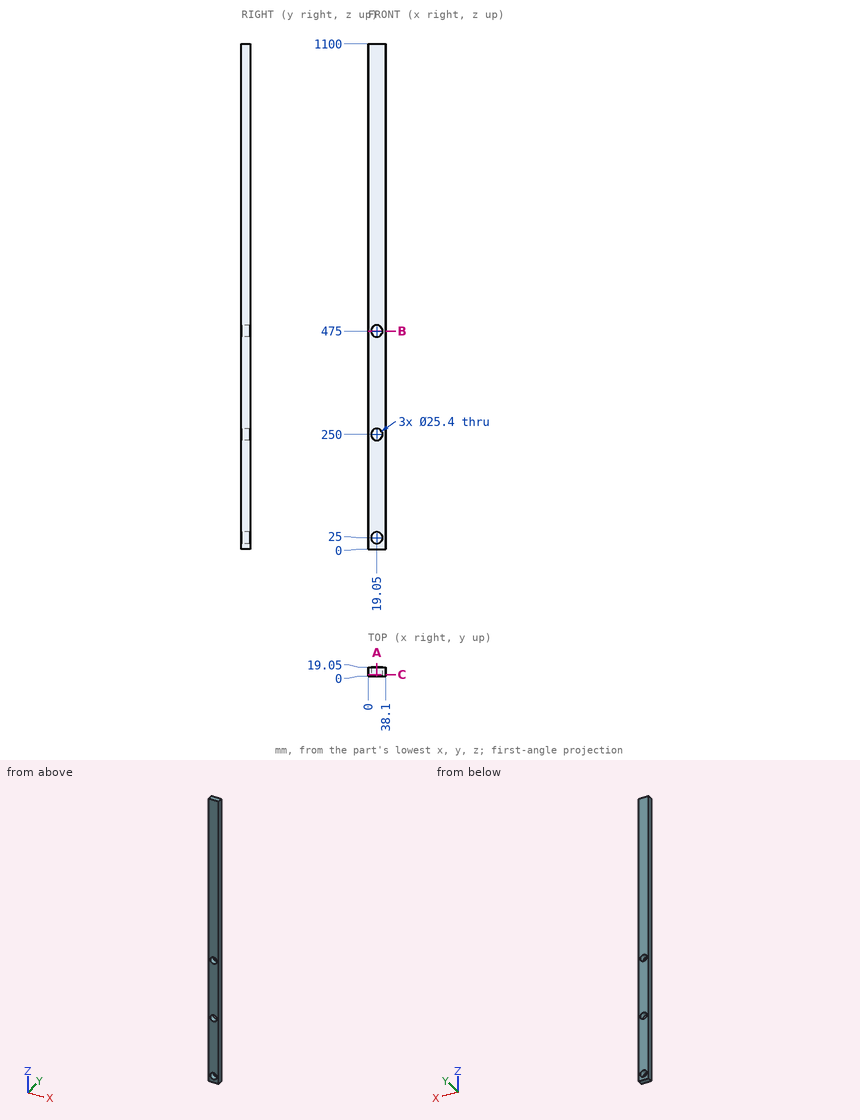
Could you check a few things on this drawing? It's one solid part, dimensions in mm from its lowest x, y, z. Round coordinates to 2 decimals unless told otherwise and drop trailing zeros. Loops run counter-clockwise (first coordinate to the right, second up) from the corner with the lowest first, then second, coordinate; pieces in that order, holes last. Notation, with made-up numbers: M 89.5,49.5 L 148.5,49.5 A23 cw 148.5,67.5 Z; hole C -32.75,42.5 d2. An arc over 180 degrees is marked long. Write each question's results on one line, items separated by ' | '. Start each with the question number.
(1) If I drill on probe 1 along Z at (x, y) = (19.05, 14.5); probe 2 along Z at (x, y) = (15, 17), over which ranges is the centre line in solid material (lowest first)? Write a range as from..to.
(2) I want a section at A-A (x = 19.05). Please give me the cut outline in (y, z).
(3) I want a section at C-C (y = 3). Please give me the cut outline in (x, z), then the cut area to 3 significant figures.
(4) I want a section at B-B (z = 475). Please give me the cut outline in (x, y).
Solved:
1) probe 1: z = 0..12.3, 37.7..237.3, 262.7..462.3, 487.7..1100 | probe 2: z = 0..12.96, 37.04..237.96, 262.04..462.96, 487.04..1100
2) outline: M 0,0 L 19.05,0 L 19.05,12.3 L 0,12.3 Z; M 0,37.7 L 19.05,37.7 L 19.05,237.3 L 0,237.3 Z; M 0,262.7 L 19.05,262.7 L 19.05,462.3 L 0,462.3 Z; M 0,487.7 L 19.05,487.7 L 19.05,1100 L 0,1100 Z
3) outline: M 0,0 L 38.1,0 L 38.1,1100 L 0,1100 Z; hole C 19.05,25 d25.4; hole C 19.05,250 d25.4; hole C 19.05,475 d25.4 | area: 40,400 mm²
4) outline: M 0,0 L 6.35,0 L 6.35,19.05 L 0,19.05 Z; M 31.75,0 L 38.1,0 L 38.1,19.05 L 31.75,19.05 Z
